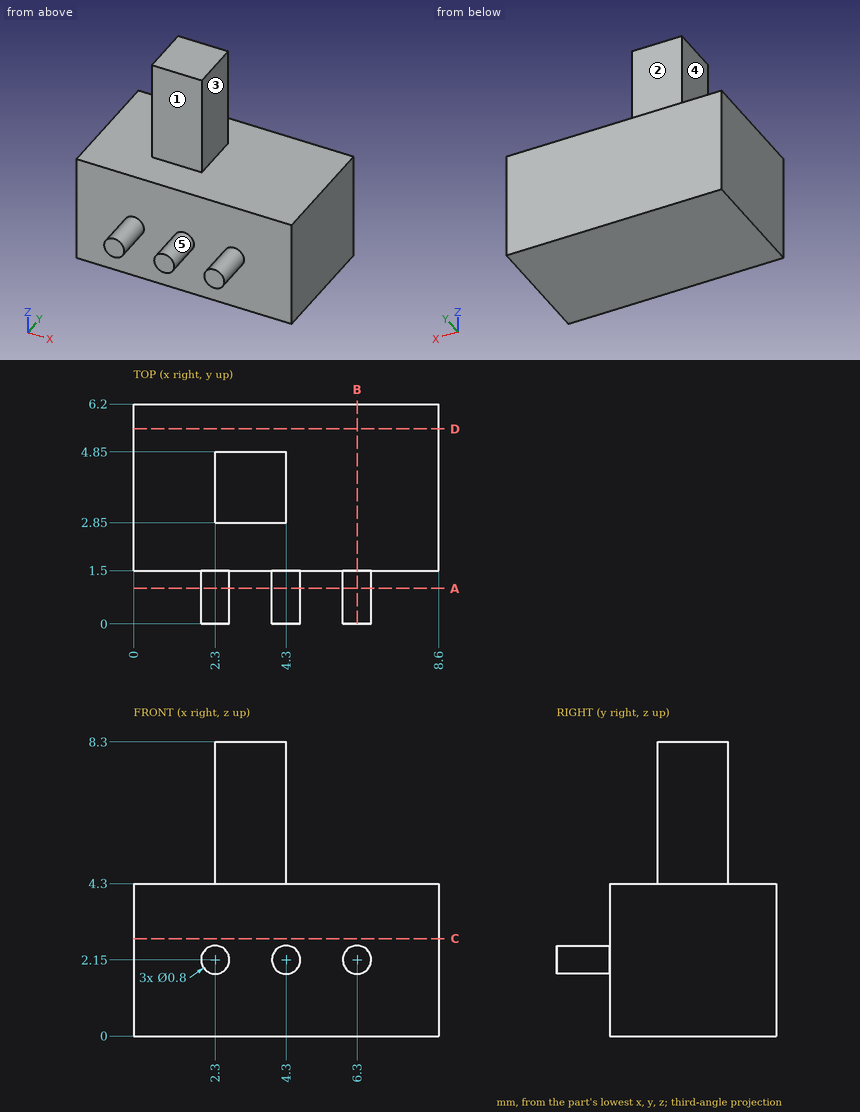
Input: dimensioned drawing with shaded views. Units: mm. Origin: part minimum x, y, z. A direction names the side the tool comes from. Give positions to 0.01 mm unless a question says otherwise; leave off trailing zeros. Order: outer loops, then holes, each group sorted by start corner. A loop starts at its lowest first (then second) coordinate and runs counter-clockwise, first axis right, second up.
(1) Material intervals for line 1 along Z through (x, y) = (5.75, 3.5); line 2 along X through (y, z) = (4, 8); line 3 along Y through (x, z) = (4, 3.75), sorted ascending.
(2) Section query A-A (y = 1). Return the cut outline in (x, z).
(3) Access query for the marked faces 1, 2, 3, 4 and 5. Directions: +Z, -Z, +X, -X, +Y, -Y. A direction counts if a zero-diameter tool reaches every point of the face in a straight line with its end or side. Return the directions, or none.
(4) Section query D-D (y = 5.5). Return the cut outline in (x, z), plus the area to 3 significant figures.
(5) Section query C-C (z = 2.75). Return the cut outline in (x, y), plus the area to 3 significant figures.
(6) Section query B-B (x = 6.3). Return the cut outline in (y, z), plus the area to 3 significant figures.
(7) Contact query for flat-ended pins moving along their axis: P1, Ø2.5, axis at x = 5.5, y = 5, coming from the +Z side; P2, Ø0.6, axis at y = 4, z = 7, coming from the +X side; P3, Ø1.6, axis at x = 3, z = 7, coming from the +Y side; P4, Ø1, axis at y = 4, z = 6.5, coming from the -X side. Output: stop coordinate, or through.
Outcome:
1. line 1: z = 0 to 4.3
1. line 2: x = 2.3 to 4.3
1. line 3: y = 1.5 to 6.2
2. outline: circle Ø0.8 at (2.3, 2.15); circle Ø0.8 at (4.3, 2.15); circle Ø0.8 at (6.3, 2.15)
3. face 1: +Z, +X, -X, -Y
3. face 2: +Z, +X, -X, +Y
3. face 3: +Z, +X, +Y, -Y
3. face 4: +Z, -X, +Y, -Y
3. face 5: -Y
4. outline: (0, 0) - (8.6, 0) - (8.6, 4.3) - (0, 4.3) - close
4. area: 37.0 mm2
5. outline: (0, 1.5) - (8.6, 1.5) - (8.6, 6.2) - (0, 6.2) - close
5. area: 40.4 mm2
6. outline: (0, 1.75) - (1.5, 1.75) - (1.5, 0) - (6.2, 0) - (6.2, 4.3) - (1.5, 4.3) - (1.5, 2.55) - (0, 2.55) - close
6. area: 21.4 mm2
7. P1: stops at z = 8.3
7. P2: stops at x = 4.3
7. P3: stops at y = 4.85
7. P4: stops at x = 2.3
